```python
from build123d import *

# Parameters (mm, degrees)
SKETCH2_W           = 1626.4
SKETCH2_H           = 914.4
BOSS_EXTRUDE1_DEPTH = 100
SHELL1_T            = -10
SKETCH3_W           = 1526.4
SKETCH3_H           = 814.4
CUT_EXTRUDE1_DEPTH  = 1868.994732327
SKETCH8_W           = 914.4
SKETCH8_H           = 42
CUT_EXTRUDE5_DEPTH  = 1869.503229861
SKETCH9_R           = 4
CUT_EXTRUDE8_DEPTH  = 1867.72663237
SKETCH10_R          = 4
CUT_EXTRUDE9_DEPTH  = 1867.442691325
SKETCH11_W          = 1610.4
SKETCH11_H          = 898.4
CUT_EXTRUDE10_DEPTH = 50
FILLET1_R           = 2.4
SKETCH13_R          = 4.5
CUT_EXTRUDE11_DEPTH = 1867.72663237


with BuildPart() as part:
    # Sketch2 → Boss-Extrude1 (new body)
    with BuildSketch(Plane(origin=(0, 0, 0), x_dir=(1, 0, 0), z_dir=(0, 1, 0))):
        with Locations((813.2, 457.2)):
            Rectangle(SKETCH2_W, SKETCH2_H)
    extrude(amount=BOSS_EXTRUDE1_DEPTH)

    # Shell1
    shell1_openings = [part.faces().sort_by_distance(p)[0] for p in [
        (813.2, 100, -457.2),
    ]]
    offset(amount=SHELL1_T, openings=shell1_openings, kind=Kind.INTERSECTION)

    # Sketch3 → Cut-Extrude1 (cut, through all)
    with BuildSketch(Plane(origin=(0, 10, 0), x_dir=(1, 0, 0), z_dir=(0, 1, 0))):
        with Locations((813.2, 457.2)):
            Rectangle(SKETCH3_W, SKETCH3_H)
    extrude(amount=-CUT_EXTRUDE1_DEPTH, mode=Mode.SUBTRACT)

    # Sketch8 → Cut-Extrude5 (cut, through all)
    with BuildSketch(Plane(origin=(1626.4, 0, 0), x_dir=(0, 0, -1), z_dir=(1, 0, 0))):
        with Locations((457.2, 79)):
            Rectangle(SKETCH8_W, SKETCH8_H)
    extrude(amount=-CUT_EXTRUDE5_DEPTH, mode=Mode.SUBTRACT)

    # Sketch9 → Cut-Extrude8 (cut, through all)
    with BuildSketch(Plane(origin=(1626.4, 0, 0), x_dir=(0, 0, -1), z_dir=(1, 0, 0))):
        with Locations((899.7, 43)):
            Circle(SKETCH9_R)
        with Locations((899.7, 26.7)):
            Circle(SKETCH9_R)
    extrude(amount=-CUT_EXTRUDE8_DEPTH, mode=Mode.SUBTRACT)

    # Sketch10 → Cut-Extrude9 (cut, through all)
    with BuildSketch(Plane(origin=(0, 10, 0), x_dir=(1, 0, 0), z_dir=(0, 1, 0))):
        with Locations(Location((30, 884.4, 0), (0, 0, 270))):
            Circle(SKETCH10_R)
        with Locations(Location((30, 30, 0), (0, 0, 270))):
            Circle(SKETCH10_R)
        with Locations(Location((1596.4, 30, 0), (0, 0, 270))):
            Circle(SKETCH10_R)
        with Locations(Location((1596.4, 884.4, 0), (0, 0, 270))):
            Circle(SKETCH10_R)
    extrude(amount=-CUT_EXTRUDE9_DEPTH, mode=Mode.SUBTRACT)

    # Sketch11 → Cut-Extrude10 (cut)
    with BuildSketch(Plane(origin=(0, 58, 0), x_dir=(1, 0, 0), z_dir=(0, 1, 0))):
        with Locations((813.2, 457.2)):
            Rectangle(SKETCH11_W, SKETCH11_H)
    extrude(amount=-CUT_EXTRUDE10_DEPTH, mode=Mode.SUBTRACT)

    # Fillet1
    fillet1_edges = [part.edges().sort_by_distance(p)[0] for p in [
        (0, 29, -914.4),
        (1626.4, 29, -914.4),
        (1626.4, 29, 0),
        (0, 29, 0),
    ]]
    fillet(fillet1_edges, radius=FILLET1_R)

    # Sketch13 → Cut-Extrude11 (cut, through all)
    with BuildSketch(Plane(origin=(1626.4, 0, 0), x_dir=(0, 0, -1), z_dir=(1, 0, 0))):
        with Locations((14.7, 43)):
            Circle(SKETCH13_R)
        with Locations((14.626959673, 26.7)):
            Circle(SKETCH13_R)
    extrude(amount=-CUT_EXTRUDE11_DEPTH, mode=Mode.SUBTRACT)


solid = part.part
```
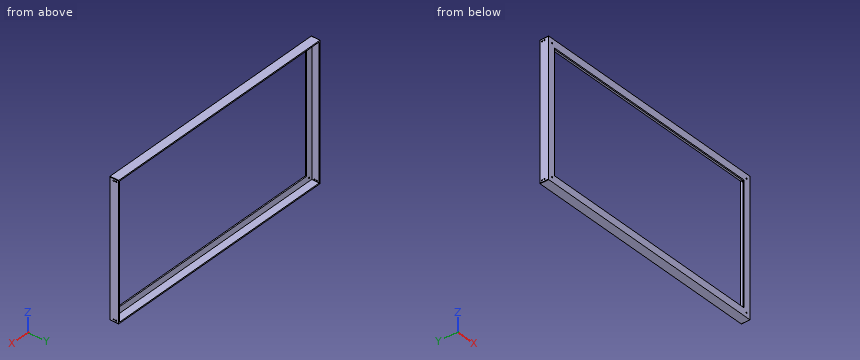
Check sheet for the modelled part. Datum: model origin and axes. Units: mm. Give positions to 0.01 mm unless a question says otherwise; leave off trailing zeros. Write each loop counter-clockwise with the first axis right and the second up, starting at its lowest first coordinate (ties: lowest second). Pieces come first, ordered by that corner, then holes. Notation, with made-up numbers: (14, 22) -> (63, 22) arc R14 ccw to (63, 31) -> close; hole circle Ø2 at (73, -7.5). An arc over 180 degrees is marked (long way). Use CSV: the item, a comma, the result in double quotes. Start each with the question number.
Q1. Cross-section at B-B on z = -105. Enter the section's corners in (x, y).
Q2. Depth check by flat-ended pin: P1, Ø3, axis at y = 25, z = -385, coming from the -X side. Enter the tip coordinate at first touch or a pass-through.
Q3. Scan lines: line 1 along X through (y, z) = (4, -30); line 2 along Z through (x, y) = (1620, 26); line 3 along Y through (x, z) = (6, -899.7). Record each from-to range of solid material in increasing order.
Q4. Cross-section at A-A on x = 1332. Enter the section's corners in (y, z), and give its area (3 significant figures).
Working result:
1,outline,"(0, 0) -> (50, 0) -> (50, 8) -> (8, 8) -> (8, 58) -> (0, 58) -> close; (1576.4, 0) -> (1626.4, 0) -> (1626.4, 58) -> (1618.4, 58) -> (1618.4, 8) -> (1576.4, 8) -> close"
2,P1,"stops at x = 0"
3,line 1,"x = 0 to 26, 34 to 1592.4, 1600.4 to 1626.4"
3,line 2,"z = -914.4 to -903.64, -895.76 to -19.07, -10.18 to 0"
3,line 3,"y = 0 to 22.7, 30.7 to 39, 47 to 58"
4,outline,"(0, -914.4) -> (58, -914.4) -> (58, -906.4) -> (8, -906.4) -> (8, -864.4) -> (0, -864.4) -> close; (0, -50) -> (8, -50) -> (8, -8) -> (58, -8) -> (58, 0) -> (0, 0) -> close"
4,area,"1,600 mm^2"
